Source: CAD feature listing. Evaluate the final solid. Frame: model axes, mm. A direction names the side the tool comes from. Round coordinates to 2 decimals unless told otherwise and drop trailing zeros. Order: outer loops, then holes, each group sorted by start corner. A loop starts at its lowest first (then second) coordinate and runs counter-clockwise, first axis right, second up. Notation, with made-up numbers: (43, 16) -> (101, 16) arc R24 cw to (101, 46) -> close; hole circle Ø6 at (79, -29.5). An arc over 180 degrees is marked (long way). Answer as CSV lines item,"result". Start each with the question number.
(1) Line query: line 1 along Z through (x, y) = (-16, -18.5); line 2 along X through (y, z) = (-17, -5); line 3 along Y through (x, z) = (-17.15, -9). Output: solid intervals per line, ascending. Write a range as from..to.
(2) Section query C-C (x = 9.5). Output: boundary loops of the cut face in (y, z), plus the area to 3 significant figures.
(3) Contact query for flat-ended pins moving along their axis: P1, Ø8, axis at y = -28.5, z = -9.5, coming from the -X side; P2, Ø1.5, axis at x = 6.5, y = -29.5, coming from the -Z side. Output: stop coordinate, or through.
(4) Set-up query: faces 5 (the flat face through (-16.152, -18, -6)), 6 (the flat face through (-11, -12.726, 1)), 7 (the flat face through (3.443, -29.328, 0.74)), 8 (the cylindrical face through (-12.13, -25.16, -6.34)). Return all of +Z, -Z, +X, -X, +Y, -Y with unobstructed straight access to the full face (end or side cutting, diameter ignored); none if empty.
(5) Section query B-B (y = -10.5). Output: boundary loops of the cut face in (x, z).
(6) Pull-direction query (Z, two-part tool) for faces 1 (the flat face through (3, -18, 1.5)), 2 (the cylindrical face through (-5.581, -3.327, 0.76)), 3 (the cylindrical face through (-17.14, -19.1, -9.72)), 4 (the flat face through (-16.4, -21.2, -12.5)); classes: +Z half, -Z half, draft (parallel to the pull), parting line (faces both ways), or undercut.
```python
from build123d import *

# Parameters (mm, degrees)
BOSS_EXTRUDE1_DEPTH = 1.5
BOSS_EXTRUDE3_DEPTH = 14
SKETCH6_R           = 1.55
CUT_EXTRUDE1_DEPTH  = 14
FILLET1_R           = 2


with BuildPart() as part:
    # Sketch1 → Boss-Extrude1 (new body)
    with BuildSketch(Plane.XY):
        Polygon((-6.151738777, -2.72550419), (24.554874692, -2.72550419), (20.100451461, -34.420372379), (-18.151738777, -22.72550419), (-18.151738777, -12.72550419), (-6.151738777, -12.72550419), align=None)
    extrude(amount=BOSS_EXTRUDE1_DEPTH)

    # Sketch5 → Boss-Extrude3 (add)
    with BuildSketch(Plane.XY.offset(1.5)):
        Polygon((-16.151738777, -23.336965553), (-11.383691284, -24.794703962), (-11.968434693, -26.707313474), (-18.151738777, -24.816887703), (-18.151738777, -12.72550419), (-16.151738777, -12.72550419), align=None)
    extrude(amount=-BOSS_EXTRUDE3_DEPTH)

    # Sketch6 → Cut-Extrude1 (cut)
    with BuildSketch(Plane(origin=(-16.151738777, 0, 0), x_dir=(0, 0, -1), z_dir=(1, 0, 0))):
        with Locations((9, -17.72550419)):
            Circle(SKETCH6_R)
    extrude(amount=-CUT_EXTRUDE1_DEPTH, mode=Mode.SUBTRACT)

    # Fillet1
    fillet1_edges = [part.edges().sort_by_distance(p)[0] for p in [
        (-18.151738777, -12.72550419, -5.5),
        (-11.383691284, -24.794703962, -6.25),
        (-18.151738777, -24.816887703, -5.5),
        (20.100451461, -34.420372379, 0.75),
        (-6.151738777, -2.72550419, 0.75),
        (24.554874692, -2.72550419, 0.75),
    ]]
    fillet(fillet1_edges, radius=FILLET1_R - 0.0001)  # a hair under: the kernel refuses the full size


solid = part.part
```
Answer block:
1,line 1,"0..1.5"
1,line 2,"-18.15..-16.15"
1,line 3,"-25.07..-19.28, -16.18..-12.99"
2,outline,"(-31.18, 0) -> (-2.73, 0) -> (-2.73, 1.5) -> (-31.18, 1.5) -> close"
2,area,"42.7 mm2"
3,P1,"x = -17.78"
3,P2,"z = 0"
4,face 5,"-Z, +X, +Y"
4,face 6,"+Z, -Z, -X, +Y"
4,face 7,"+Z, -Z, -Y"
4,face 8,"-Z, +X"
5,outline,"(-6.15, 0) -> (23.46, 0) -> (23.46, 1.5) -> (-6.15, 1.5) -> close"
6,face 1,"+Z half"
6,face 2,"draft"
6,face 3,"undercut"
6,face 4,"-Z half"
